from build123d import *

# Parameters (mm, degrees)
SKETCH1_R              = 4
BOSS_EXTRUDE1_DEPTH    = 45
SKETCH2_W              = 50.339144224
SKETCH2_H              = 25
CUT_EXTRUDE1_DEPTH     = 20
SKETCH3_R              = 4
BOSS_EXTRUDE2_DEPTH    = 5
CUT_EXTRUDE2_REACH     = 88.493
SKETCH4_W              = 77.888808367
SKETCH4_H              = 40
SKETCH5_W              = 18
SKETCH5_H              = 15
CUT_EXTRUDE3_DEPTH     = 84.739178405
FILLET1_R              = 4
LPATTERN1_COUNT        = 3
LPATTERN1_PITCH        = 30
FILLET1_OF_LPATTERN1_R = 4
SHELL1_START           = 2
SHELL1_DEPTH           = 41
SHELL1_START_2         = -3
SHELL1_2_OUTLINE_R     = 2
SHELL1_2_DEPTH         = 51


# Read off the part's stored shape, not the designer's step: Shell1
with BuildPart() as part:
    # Sketch1 → Boss-Extrude1 (new body)
    with BuildSketch(Plane(origin=(0, 0, 0), x_dir=(1, 0, 0), z_dir=(0, 1, 0))):
        with BuildLine():
            Line((-53.5, -12.5), (53.5, -12.5))
            ThreePointArc((53.5, -12.5), (66, 0), (53.5, 12.5))
            Line((53.5, 12.5), (-53.5, 12.5))
            ThreePointArc((-53.5, 12.5), (-66, 0), (-53.5, -12.5))
        make_face()
        with Locations(Location((53.5, 0, 0), (0, 0, 90))):
            Circle(SKETCH1_R, mode=Mode.SUBTRACT)
    extrude(amount=BOSS_EXTRUDE1_DEPTH)

    # Sketch2 → Cut-Extrude1 (cut, symmetric)
    with BuildSketch(Plane(origin=(0, 22.5, 0), x_dir=(1, 0, 0), z_dir=(0, 1, 0))):
        with Locations((53.5, 0)):
            Rectangle(SKETCH2_W, SKETCH2_H)
    extrude(amount=CUT_EXTRUDE1_DEPTH, both=True, mode=Mode.SUBTRACT)

    # Sketch3 → Boss-Extrude2 (add, symmetric)
    with BuildSketch(Plane(origin=(0, 45, 0), x_dir=(1, 0, 0), z_dir=(0, 1, 0))):
        with Locations(Location((-53.5, 0, 0), (0, 0, 270))):
            Circle(SKETCH3_R)
    boss_extrude2 = extrude(amount=BOSS_EXTRUDE2_DEPTH, both=True)

    # Mirror1: Boss-Extrude2 across plane
    add(boss_extrude2.mirror(Plane.ZX.offset(22.5)))

    # Sketch4 → Cut-Extrude2 (cut, up to next)
    with BuildSketch(Plane(origin=(0, 0, -12.5), x_dir=(-1, 0, 0), z_dir=(0, 0, -1)), mode=Mode.PRIVATE) as cut_extrude2_sk1:
        with Locations((10.613976295, 22.5)):
            Rectangle(SKETCH4_W, SKETCH4_H)
    cut_extrude2_tool1 = extrude(cut_extrude2_sk1.sketch, amount=-CUT_EXTRUDE2_REACH, mode=Mode.PRIVATE) & part.part
    add(cut_extrude2_tool1.solids().sort_by_distance((-10.613976, 22.5, -12.5))[0], mode=Mode.SUBTRACT)

    # Sketch5 → Cut-Extrude3 (cut, through all)
    with BuildSketch(Plane(origin=(0, 45, 0), x_dir=(1, 0, 0), z_dir=(0, 1, 0))):
        with Locations((-32.941043084, 0)):
            Rectangle(SKETCH5_W, SKETCH5_H)
    cut_extrude3 = extrude(amount=-CUT_EXTRUDE3_DEPTH, mode=Mode.SUBTRACT)

    # Fillet1
    fillet1_edges = [part.edges().sort_by_distance(p)[0] for p in [
        (-41.941043084, 1.25, 7.5),
        (-41.941043084, 1.25, -7.5),
        (-23.941043084, 1.25, -7.5),
        (-23.941043084, 1.25, 7.5),
        (-41.941043084, 43.75, 7.5),
        (-41.941043084, 43.75, -7.5),
        (-23.941043084, 43.75, -7.5),
        (-23.941043084, 43.75, 7.5),
    ]]
    fillet(fillet1_edges, radius=FILLET1_R)

    # LPattern1: Cut-Extrude3 ×3
    with Locations(*[(i * LPATTERN1_PITCH, 0, 0) for i in range(1, LPATTERN1_COUNT)]):
        add(cut_extrude3, mode=Mode.SUBTRACT)

    # Fillet1 of LPattern1
    fillet1_of_lpattern1_edges = [part.edges().sort_by_distance(p)[0] for p in [
        (-11.941043084, 1.25, 7.5),
        (-11.941043084, 1.25, -7.5),
        (6.058956916, 1.25, -7.5),
        (6.058956916, 1.25, 7.5),
        (-11.941043084, 43.75, 7.5),
        (-11.941043084, 43.75, -7.5),
        (6.058956916, 43.75, -7.5),
        (6.058956916, 43.75, 7.5),
        (18.058956916, 1.25, 7.5),
        (18.058956916, 1.25, -7.5),
        (36.058956916, 1.25, -7.5),
        (36.058956916, 1.25, 7.5),
        (18.058956916, 43.75, 7.5),
        (18.058956916, 43.75, -7.5),
        (36.058956916, 43.75, -7.5),
        (36.058956916, 43.75, 7.5),
    ]]
    fillet(fillet1_of_lpattern1_edges, radius=FILLET1_OF_LPATTERN1_R)

    # Shell1 outline → Shell1 (cut)
    with BuildSketch(Plane(origin=(0, 0, 0), x_dir=(1, 0, 0), z_dir=(0, 1, 0)).offset(SHELL1_START)):
        with BuildLine():
            Line((-49.558380479, -10.5), (-49.558380479, 10.5))
            Line((-49.558380479, 10.5), (-53.5, 10.5))
            ThreePointArc((-53.5, 10.5), (-64, 0), (-53.5, -10.5))
            Line((-53.5, -10.5), (-49.558380479, -10.5))
        make_face()
    extrude(amount=SHELL1_DEPTH, mode=Mode.SUBTRACT)

    # Shell1 2 outline → Shell1 2 (cut)
    with BuildSketch(Plane(origin=(0, 0, 0), x_dir=(1, 0, 0), z_dir=(0, 1, 0)).offset(SHELL1_START_2)):
        with Locations((-53.5, 0)):
            Circle(SHELL1_2_OUTLINE_R)
    extrude(amount=SHELL1_2_DEPTH, mode=Mode.SUBTRACT)


solid = part.part
Could you check a few things on this model? Use its own coordinates, in mm. A direction names the side the tool comes from. Give positions to 0.01 mm unless a question says otherwise; leave off trailing zeros. Order: outer loops, then holes, each group sorted by start corner. A loop starts at its lowest first (then second) coordinate and runs counter-clockwise, first axis right, second up.
Item 1: If we section it at D-D, the plane z = -5.25: Count the separate pieces of the cut face and the enclosed holes in it, plus the area to 3 significant figures.
Item 2: I need wall thicknesses on line 1 (X direction, y = 44.3, z = 0); line 2 (Z direction, x = 53.5, y = 1.4); line 3 (Y direction, x = 36, z = 11.5). Which ranges of each line are inside material? Lowest first, please.
Item 3: If we mould it in two halves opening along X, with no side actions, what happens to faces 1 (the face through (-1, 45, -9)), 2 (the face through (18.059, 44, 0)), 3 (the face through (6.059, 44, 0)), 4 (the face through (-66, 22, 0))? For each: pulls with the +X half, pulls with the -X half, needs draft (parallel to the pull), parting line crosses it, or undercut.
Item 4: If we section it at A-A, the plane x = 15: Write out the boundary of the cut face in (y, z), plus the area to 3 significant figures.
Item 5: For faces 5 (the face through (-54, 48, 0)), 6 (the face through (-53, 50, 0)), 7 (the face through (-3, 1, -7.5)), which set-ups out of +Z, -Z, +X, -X, +Y, -Y let a thin tool reach every point of the face, with its end or its side?
Item 6: If we section it at C-C, the plane y = 10: Write out the boundary of the cut face in (x, z).
Item 7: If we section it at B-B, the plane x = 30.5: Write out the boundary of the cut face in (y, z), plus the area to 3 significant figures.
Item 8: I'm going to push flat-ended pins straight in: pin 1 (4.5 mm diameter, centred on x = -60, z = 5, fed in from +Y); pin 2 (1.2 mm diameter, centred on y = 43, z = -1, fed in from -X); pin 3 (4 mm diameter, centred on y = 24, z = -7, fed in from +X); pin 4 (0.8 mm diameter, centred on y = 1.5, z = 0.5, fed in from +X). Where does each tip first touch, or does it pass through?
Values:
1. separate pieces: 7
1. enclosed holes: 0
1. area: 468 mm2
2. line 1: x = -66 to -55.5, -51.5 to -41.94, -23.94 to -11.94, 6.06 to 18.06, 36.06 to 49.5, 57.5 to 66
2. line 2: z = -12.5 to -4, 4 to 12.5
2. line 3: y = 0 to 2.5, 42.5 to 45
3. face 1: needs draft
3. face 2: undercut
3. face 3: undercut
3. face 4: pulls with the -X half
4. outline: (0, -12.5) - (2.5, -12.5) - (2.5, 12.5) - (0, 12.5) - close; (42.5, -12.5) - (45, -12.5) - (45, 12.5) - (42.5, 12.5) - close
4. area: 125 mm2
5. face 5: none
5. face 6: +Z, -Z, +X, -X, +Y
5. face 7: +Y, -Y
6. outline: (-53.5, -12.5) - (-49.56, -12.5) - (-49.56, -10.5) - (-53.5, -10.5) arc R10.5 cw to (-53.5, 10.5) - (-49.56, 10.5) - (-49.56, 12.5) - (-53.5, 12.5) arc R12.5 ccw to start
7. outline: (0, -12.5) - (2.5, -12.5) - (2.5, -7.5) - (0, -7.5) - close; (0, 7.5) - (2.5, 7.5) - (2.5, 12.5) - (0, 12.5) - close; (42.5, -12.5) - (45, -12.5) - (45, -7.5) - (42.5, -7.5) - close; (42.5, 7.5) - (45, 7.5) - (45, 12.5) - (42.5, 12.5) - close
7. area: 50.0 mm2
8. pin 1: stops at y = 45
8. pin 2: stops at x = -65.99
8. pin 3: stops at x = -58.91
8. pin 4: stops at x = 66
